Verification items for the finished model (mm, model axes). A direction names the side the tool comes from. Round coordinates to 2 decimals unless told otherwise and drop trailing zeros. Order: outer loops, then holes, each group sorted by start corner. A loop starts at its lowest first (then second) coordinate and runs counter-clockwise, first axis right, second up. Notation, with made-up numbers: (-2.5, 40.25) -> (52.5, 40.25) arc R23 ccw to (52.5, 74.25) -> close; hole circle Ø2 at (8.5, 80). An arc over 180 degrees is marked (long way). Return JSON: item names as keys, results as strings. Group by question number.
1) Scan lines: L1, parallel to Y at x = 1.75, z = 0.3; L2, parallel to Y at x = 3, z = 2.6; L3, parallel to X at y = 13.5, z = 1.2. Record each from-to range of solid material in increasing order.
2) Section check C-C on z = 1.95. Enter the section's corners in (x, y).
3) Section check B-B on x = -0.5. Enter the section's corners in (y, z), plus the area to 3 significant figures.
4) Depth check by flat-ended pin: pin 1 (1.5 mm diameter, centred on y = -6, z = 2, fed in from +X). Enter the tip coordinate at first touch or a pass-through.
5) Section check D-D on y = -7.5. Enter the section's corners in (x, z).
6) Draft check along X on faces 1 (the flat face through (0, -11.25, 1)), 2 (the cylindrical face through (-3.9, -12.9, 1.5)), 3 (the flat face through (0, 16.4, 1)), 4 (the flat face through (6, 0.2, 1.5)). Enter one of: pulls with the +X half, pulls with the -X half, needs draft (parallel to the pull), parting line crosses it, or undercut.
7) Tool access check on faces 5 (the flat face through (-1, 0, 0)), 6 (the flat face through (0, 11.25, 1)). Record the directions out of +Z, -Z, +X, -X, +Y, -Y that give a thin tool (end or side, any length) a straight path to the whole face; none if there is none.
8) Section check A-A on y = 12.9. Enter the section's corners in (x, z), plus the area to 3 significant figures.
```python
from build123d import *

# Parameters (mm, degrees)
F0_W     = 13
F0_H     = 32.8
F1_DEPTH = 3
F3_DEPTH = 32.801


with BuildPart() as f1:
    # F0 (on Top) → F1 (new body)
    with BuildSketch(Plane.XY):
        with Locations((1.5, 0)):
            Rectangle(F0_W, F0_H)
        with BuildLine():
            Line((2.25, -14.55), (-2.25, -14.55))
            ThreePointArc((-2.25, -14.55), (-3.9, -12.9), (-2.25, -11.25))
            Line((-2.25, -11.25), (2.25, -11.25))
            ThreePointArc((2.25, -11.25), (3.9, -12.9), (2.25, -14.55))
        make_face(mode=Mode.SUBTRACT)
        with BuildLine():
            ThreePointArc((-2.25, 11.25), (-3.9, 12.9), (-2.25, 14.55))
            Line((-2.25, 14.55), (2.25, 14.55))
            ThreePointArc((2.25, 14.55), (3.9, 12.9), (2.25, 11.25))
            Line((2.25, 11.25), (-2.25, 11.25))
        make_face(mode=Mode.SUBTRACT)
    extrude(amount=F1_DEPTH)

    # F2 (on face) → F3 (cut, through all)
    with BuildSketch(Plane(origin=(0, 16.4, 0), x_dir=(-1, 0, 0), z_dir=(0, 1, 0))):
        Polygon((-4, 0), (-8, 3), (-8, 0), align=None)
    extrude(amount=-F3_DEPTH, mode=Mode.SUBTRACT)


solid = f1.part
```
Check result:
{
 "1": {"L1": "-16.4 to -14.55, -11.25 to 11.25, 14.55 to 16.4", "L2": "-16.4 to -14.37, -11.43 to 11.43, 14.37 to 16.4", "L3": "-5 to -3.79, 3.79 to 5.6"},
 "2": {"outline": "(-5, -16.4) -> (6.6, -16.4) -> (6.6, 16.4) -> (-5, 16.4) -> close; hole (-2.25, -14.55) -> (2.25, -14.55) arc R1.65 ccw to (2.25, -11.25) -> (-2.25, -11.25) arc R1.65 ccw to start; hole (-2.25, 11.25) -> (2.25, 11.25) arc R1.65 ccw to (2.25, 14.55) -> (-2.25, 14.55) arc R1.65 ccw to start"},
 "3": {"outline": "(-16.4, 0) -> (-14.55, 0) -> (-14.55, 3) -> (-16.4, 3) -> close; (-11.25, 0) -> (11.25, 0) -> (11.25, 3) -> (-11.25, 3) -> close; (14.55, 0) -> (16.4, 0) -> (16.4, 3) -> (14.55, 3) -> close", "area": "78.6 mm^2"},
 "4": {"pin 1": "x = 7.67"},
 "5": {"outline": "(-5, 0) -> (4, 0) -> (8, 3) -> (-5, 3) -> close"},
 "6": {"face 1": "undercut", "face 2": "undercut", "face 3": "needs draft", "face 4": "pulls with the +X half"},
 "7": {"face 5": "-Z, +X, -X, +Y, -Y", "face 6": "+Z, -Z"},
 "8": {"outline": "(-5, 0) -> (-3.9, 0) -> (-3.9, 3) -> (-5, 3) -> close; (3.9, 0) -> (4, 0) -> (8, 3) -> (3.9, 3) -> close", "area": "9.60 mm^2"}
}
